Could you check a few things on this model? Use its own coordinates, in mm. A direction names the side the tool comes from. Give positions to 0.01 mm unless a question says otherwise; leave off trailing zeros. Loops run counter-clockwise (first coordinate to the right, second up) from the corner with the lowest first, then second, coordinate; pieces in that order, holes last. Notation, with made-up numbers: (-10.5, -11.75) - (16.5, -11.75) arc R21 ccw to (16.5, 22.25) - close; hole circle Ø5 at (-1.75, 10.25). An arc over 180 degrees is marked (long way). One line per item, written item: value. Start each with the question number.
Q1. I want a section at A-A (y = 16.41). Please give me the cut outline in (x, z).
Q2. I want a section at B-B (z = 1.45). Please give me the cut outline in (x, y).
Q3. I want a section at C-C (x = 14). Please give me the cut outline in (y, z).
Q4. I want a section at D-D (x = 2.25). Please give me the cut outline in (y, z).
Q5. I'm going to push flat-ended pins straight in: P1, Ø3, axis at x = 14, y = 16.41, coming from the +Z side; P2, Ø1.2, axis at x = 2, z = 2.5, coming from the -Y side; P3, Ø1.2, axis at y = -2, z = 2, coming from the -X side. Where does each tip first touch, or does it pass through?
Q6. If we mould it in two halves opening along Y, with no side actions, what happens to faces 4 (the face through (14.055, -4.572, 1.972)), 5 (the face through (0, 8, 2)), 6 (the face through (11.5, 16.5, 2))? For each: released by +Y, released by -Y, zero draft, split by the parting line, or undercut.
Q7. If I drill on line 1 (Y direction, x = 12, z = 0.35); line 2 (Y direction, x = 14, z = 1.3); line 3 (X direction, y = 18.25, z = 0.2), over which ranges is the centre line in solid material (lowest first)? Write a range as from..to.
Q8. For faces 1 (the face through (22.956, -1.3, 2.028)), 2 (the face through (4, 19, 2)), 3 (the face through (4, -3, 2)), which set-ups out of +Z, -Z, +X, -X, +Y, -Y let a thin tool reach every point of the face, with its end or its side?
```python
from build123d import *

# Parameters (mm, degrees)
SKETCH_1_R      = 2.5
EXTRUDE_1_DEPTH = 4
FILLET_1_R      = 5


with BuildPart() as part:
    # ｽｹｯﾁ1 → ﾎﾞｽ - 押し出し1 (new body)
    with BuildSketch(Plane.XY):
        Polygon((0, 15), (0, 0), (4, 0), (4, -6), (8.110763801, -6), (24, -2.18322685), (24, 22), (4, 22), (4, 15), align=None)
        with Locations((14, 16.41)):
            Circle(SKETCH_1_R, mode=Mode.SUBTRACT)
    extrude(amount=EXTRUDE_1_DEPTH)

    # ﾌｨﾚｯﾄ1
    fillet_1_edges = [part.edges().sort_by_distance(p)[0] for p in [
        (24, 22, 2),
        (24, -2.18322685, 2),
    ]]
    fillet(fillet_1_edges, radius=FILLET_1_R)


solid = part.part
```
Worked answers:
1. outline: (4, 0) - (11.5, 0) - (11.5, 4) - (4, 4) - close; (16.5, 0) - (24, 0) - (24, 4) - (16.5, 4) - close
2. outline: (0, 0) - (4, 0) - (4, -6) - (8.11, -6) - (20.17, -3.1) arc R5 ccw to (24, 1.76) - (24, 17) arc R5 ccw to (19, 22) - (4, 22) - (4, 15) - (0, 15) - close; hole circle Ø5 at (14, 16.41)
3. outline: (-4.59, 0) - (13.91, 0) - (13.91, 4) - (-4.59, 4) - close; (18.91, 0) - (22, 0) - (22, 4) - (18.91, 4) - close
4. outline: (0, 0) - (15, 0) - (15, 4) - (0, 4) - close
5. P1: passes through
5. P2: stops at y = 0
5. P3: stops at x = 4
6. face 4: released by -Y
6. face 5: zero draft
6. face 6: undercut
7. line 1: y = -5.07..14.91, 17.91..22
7. line 2: y = -4.59..13.91, 18.91..22
7. line 3: x = 4..12.31, 15.69..23.84
8. face 1: +Z, -Z, +X, -Y
8. face 2: +Z, -Z, -X, +Y
8. face 3: +Z, -Z, -X, -Y
